For this review, take the finished solid that the model builds, in its own axes (mm). A direction names the side the tool comes from. Coordinates: 2 decimals unless noted, no trailing zeros. Loops run counter-clockwise (first coordinate to the right, second up) from the corner with the lowest first, then second, coordinate; pieces in that order, holes last. Notation, with made-up numbers: (-10.75, 20.5) - (31.25, 20.5) arc R27 cw to (31.25, 53.5) - close; hole circle Ø2 at (-16, 2.25). An arc over 180 degrees is marked (long way). One line per item, written item: value. Start each with the question number.
1. To check wall thickness, follow line 1 (Y direction, x = -30.5, z = 38); line 2 (X direction, y = 25, z = 92); line 3 (X direction, y = 19, z = 75.5). State the ranges of each line that lie inside material, in increasing order. Write a range as from..to.
2. Take a section at C-C, the plane z = 57. State the section outline as (x, y) points, and give its area (3 significant figures).
3. Take a section at A-A, the plane y = 15. State the section outline as (x, z) points, and give its area (3 significant figures).
4. Take a section at D-D, the plane x = 0. State the section outline as (y, z) points.
5. Insertion check: pin 1 (23.5 mm diameter, centred on x = 41.5, y = 26.5, fed in from +Z); pin 2 (6.5 mm diameter, centred on x = -35, z = 56.5, fed in from +Y); pin 3 (1.5 mm diameter, centred on y = 17.5, z = 102.5, fed in from -X); pin 4 (10 mm diameter, centred on x = 4.5, y = 7.5, fed in from -Z). Each pin has a flat end and moves straight along its axis. Give the tip position at first contact, or say it passes through.
6. Take a section at B-B, the plane x = -35. State the section outline as (y, z) points, and give its area (3 significant figures).
7. The part is to be moulded in two halves that separate along X. For faces 4 (the face through (-1, -8, 0)), 5 (the face through (-0.559, 12.706, 64.389)), 6 (the face through (29.21, 25, 77)), say which applies: released by +X, released by -X, zero draft, split by the parting line, or undercut.
8. For faces 1 (the face through (-40, 12.7, 77)), 2 (the face through (40, 12.7, 77)), 3 (the face through (50.8, -9, 63)), list the 3-axis set-ups (+Z, -Z, +X, -X, +Y, -Y) from which the entire face can be reached by the end or side of a thin tool; tool diameter is ignored.
```python
from build123d import *

# Parameters (mm, degrees)
F0_W     = 101.6
F0_H     = 76.2
F1_DEPTH = 127
F3_DEPTH = 127.001
F4_W     = 21.5898367196
F4_H     = 25.4
F5_DEPTH = 101.6


with BuildPart() as f1:
    # F0 (on Top) → F1 (new body)
    with BuildSketch(Plane.XY):
        Rectangle(F0_W, F0_H)
    extrude(amount=F1_DEPTH)

    # F2 (on face) → F3 (cut, through all)
    with BuildSketch(Plane.XY.offset(127)):
        with BuildLine():
            ThreePointArc((-25.4, 38.1), (0, 12.7), (25.4, 38.1))
            Line((25.4, 38.1), (-25.4, 38.1))
        make_face()
    extrude(amount=-F3_DEPTH, mode=Mode.SUBTRACT)

    # F4 (on face) → F5 (cut)
    with BuildSketch(Plane.XY.offset(127)):
        with Locations((-40.0050816402, 25.4)):
            Rectangle(F4_W, F4_H)
        with Locations((40.0050816402, 25.4)):
            Rectangle(F4_W, F4_H)
    extrude(amount=-F5_DEPTH, mode=Mode.SUBTRACT)


solid = f1.part
```
Solutions:
1. line 1: -38.1..12.7
1. line 2: -29.21..-21.76, 21.76..29.21
1. line 3: -29.21..-16.74, 16.74..29.21
2. outline: (-50.8, -38.1) - (50.8, -38.1) - (50.8, 12.7) - (29.21, 12.7) - (29.21, 38.1) - (25.4, 38.1) arc R25.4 cw to (-25.4, 38.1) - (-29.21, 38.1) - (-29.21, 12.7) - (-50.8, 12.7) - close
2. area: 5,630 mm2
3. outline: (-50.8, 0) - (-10.56, 0) - (-10.56, 127) - (-29.21, 127) - (-29.21, 25.4) - (-50.8, 25.4) - close; (10.56, 0) - (50.8, 0) - (50.8, 25.4) - (29.21, 25.4) - (29.21, 127) - (10.56, 127) - close
3. area: 5,830 mm2
4. outline: (-38.1, 0) - (12.7, 0) - (12.7, 127) - (-38.1, 127) - close
5. pin 1: z = 25.4
5. pin 2: y = 12.7
5. pin 3: x = -29.21
5. pin 4: z = 0
6. outline: (-38.1, 0) - (38.1, 0) - (38.1, 25.4) - (12.7, 25.4) - (12.7, 127) - (-38.1, 127) - close
6. area: 7,100 mm2
7. face 4: zero draft
7. face 5: undercut
7. face 6: released by +X
8. face 1: +Z, -X, +Y
8. face 2: +Z, +X, +Y
8. face 3: +Z, -Z, +X, +Y, -Y
